Could you check a few things on this model? Use its own coordinates, in mm. Face numbers are marked on the shaded views. A direction names the side the tool comes from. Give positions to 0.01 mm unless a question says otherwise; leave off trailing zeros. Write each loop counter-clockwise with the first axis right and the second up, starting at its lowest first coordinate (ties: lowest second). Pieces come first, ordered by that corner, then holes. Notation, with made-up numbers: (60, 89) - (93, 89) arc R33 cw to (93, 121) - close; hole circle Ø8 at (36, 50.5). An arc over 180 degrees is marked (long way). Write item = value, one per line.
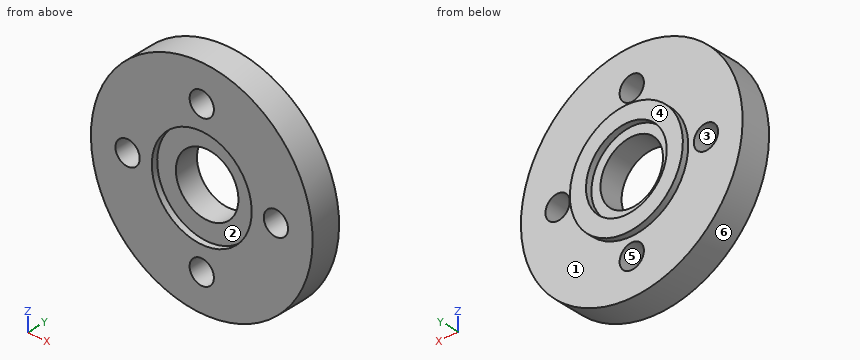
from build123d import *

# Parameters (mm, degrees)
CROQUIS_BASE_R             = 10.982321859
SALIENTE_EXTRUIR1_DEPTH    = 2.95
CORTAR_EXTRUIR1_DEPTH      = 16.809025486
CORTAR_EXTRUIR1_DEPTH_BACK = 16.809025486
CROQUIS_BASE_3_R           = 3
CROQUIS_BASE_3_R_2         = 1.202825727
CROQUIS_BASE_4_R           = 4.95
CORTAR_EXTRUIR2_DEPTH      = 0.6
CROQUIS2_R                 = 5.6
SALIENTE_EXTRUIR2_DEPTH    = 0.6
CROQUIS3_R                 = 3.1
CORTAR_EXTRUIR3_DEPTH      = 16.931895268
CROQUIS3_3_R               = 4
CORTAR_EXTRUIR4_DEPTH      = 0.6


with BuildPart() as part:
    # Croquis base → Saliente-Extruir1 (new body)
    with BuildSketch(Plane(origin=(0, 0, 0), x_dir=(1, 0, 0), z_dir=(0, 1, 0))):
        with Locations(Location((0, 0, 0), (0, 0, 270))):
            Circle(CROQUIS_BASE_R)
    extrude(amount=SALIENTE_EXTRUIR1_DEPTH)

    # Croquis base_3 → Cortar-Extruir1 (cut, two sides: drawn at the far end of the back side and taken through both)
    with BuildSketch(Plane(origin=(0, 0, 0), x_dir=(1, 0, 0), z_dir=(0, 1, 0)).offset(-CORTAR_EXTRUIR1_DEPTH_BACK)):
        with Locations(Location((0, 0, 0), (0, 0, 270))):
            Circle(CROQUIS_BASE_3_R)
        with Locations(Location((-7.35, 0, 0), (0, 0, 270))):
            Circle(CROQUIS_BASE_3_R_2)
        with Locations(Location((0, 7.35, 0), (0, 0, 270))):
            Circle(CROQUIS_BASE_3_R_2)
        with Locations(Location((7.35, 0, 0), (0, 0, 270))):
            Circle(CROQUIS_BASE_3_R_2)
        with Locations(Location((0, -7.35, 0), (0, 0, 270))):
            Circle(CROQUIS_BASE_3_R_2)
    extrude(amount=CORTAR_EXTRUIR1_DEPTH + CORTAR_EXTRUIR1_DEPTH_BACK, mode=Mode.SUBTRACT)

    # Croquis base_4 → Cortar-Extruir2 (cut)
    with BuildSketch(Plane(origin=(0, 0, 0), x_dir=(1, 0, 0), z_dir=(0, 1, 0))):
        with Locations(Location((0, 0, 0), (0, 0, 270))):
            Circle(CROQUIS_BASE_4_R)
    extrude(amount=CORTAR_EXTRUIR2_DEPTH, mode=Mode.SUBTRACT)

    # Croquis2 → Saliente-Extruir2 (add)
    with BuildSketch(Plane(origin=(0, 2.95, 0), x_dir=(1, 0, 0), z_dir=(0, 1, 0))):
        with Locations(Location((0, 0, 0), (0, 0, 270))):
            Circle(CROQUIS2_R)
    extrude(amount=SALIENTE_EXTRUIR2_DEPTH)

    # Croquis3 → Cortar-Extruir3 (cut, through all)
    with BuildSketch(Plane(origin=(0, 3.55, 0), x_dir=(1, 0, 0), z_dir=(0, 1, 0))):
        with Locations(Location((0, 0, 0), (0, 0, 270))):
            Circle(CROQUIS3_R)
    extrude(amount=-CORTAR_EXTRUIR3_DEPTH, mode=Mode.SUBTRACT)

    # Croquis3_3 → Cortar-Extruir4 (cut)
    with BuildSketch(Plane(origin=(0, 3.55, 0), x_dir=(1, 0, 0), z_dir=(0, 1, 0))):
        with Locations(Location((0, 0, 0), (0, 0, 270))):
            Circle(CROQUIS3_3_R)
    extrude(amount=-CORTAR_EXTRUIR4_DEPTH, mode=Mode.SUBTRACT)


solid = part.part
1. If we section it at D-D, the plane z = 7.35: Please give me the cut outline in (x, y), and give its area (3 significant figures).
Filled sheet:
outline = (-8.16, 0) - (-1.2, 0) - (-1.2, 2.95) - (-8.16, 2.95) - close; (1.2, 0) - (8.16, 0) - (8.16, 2.95) - (1.2, 2.95) - close
area = 41.0 mm2
2. I need wall thicknesses on line 1 (X direction, y = 1.25, z = 0); line 2 (X direction, y = 0.3, z = 0); line 3 (Y direction, x = -5.5, z = -2.5). Which ranges of each line are inside material? Lowest first, please.
Filled sheet:
line_1 = -10.98 to -8.55, -6.15 to -3.1, 3.1 to 6.15, 8.55 to 10.98
line_2 = -10.98 to -8.55, -6.15 to -4.95, 4.95 to 6.15, 8.55 to 10.98
line_3 = 0 to 2.95
3. Which directions (+Z, -Z, +X, -X, +Y, -Y) give clear straight access to the entire face, cutting with the end or side of a thin tool? Please do the marked faces 1, 2 and 3.
Filled sheet:
face_1 = +Y
face_2 = -Y
face_3 = +Y, -Y
4. Thinking about a two-plate mould opening in X: for the marked faces 4, 5 and 6, which applies, pulls with the +X half, pulls with the -X half, needs draft (parallel to the pull), parting line crosses it, or undercut?
Filled sheet:
face_4 = needs draft
face_5 = undercut
face_6 = parting line crosses it
5. For pin 1 (3 mm diameter, centred on x = -1, z = -2.5, fed in from -Y); pin 2 (3 mm diameter, centred on x = -7.35, z = 0, fed in from +Y); pin 3 (1 mm diameter, centred on x = -5.5, y = 2, fed in from -Z), each with a flat end and sliding along its axis, tell me the tip position at first contact or that it passes through.
Filled sheet:
pin_1 = 0.6
pin_2 = 2.95
pin_3 = -9.78
6. If we section it at C-C, the plane y = 2.3: Please give me the cut outline in (x, z), and give its area (3 significant figures).
Filled sheet:
outline = circle Ø21.96 at (0, 0); hole circle Ø2.41 at (-7.35, 0); hole circle Ø6.2 at (0, 0); hole circle Ø2.41 at (0, -7.35); hole circle Ø2.41 at (0, 7.35); hole circle Ø2.41 at (7.35, 0)
area = 331 mm2
7. If we section it at B-B, the plane z = 0: Please give me the cut outline in (x, y), and give its area (3 significant figures).
Filled sheet:
outline = (-10.98, 0) - (-8.55, 0) - (-8.55, 2.95) - (-10.98, 2.95) - close; (-6.15, 0) - (-4.95, 0) - (-4.95, 0.6) - (-3.1, 0.6) - (-3.1, 2.95) - (-4, 2.95) - (-4, 3.55) - (-5.6, 3.55) - (-5.6, 2.95) - (-6.15, 2.95) - close; (3.1, 0.6) - (4.95, 0.6) - (4.95, 0) - (6.15, 0) - (6.15, 2.95) - (5.6, 2.95) - (5.6, 3.55) - (4, 3.55) - (4, 2.95) - (3.1, 2.95) - close; (8.55, 0) - (10.98, 0) - (10.98, 2.95) - (8.55, 2.95) - close
area = 32.0 mm2
8. If we section it at A-A, the plane x = 0: Please give me the cut outline in (y, z).
Filled sheet:
outline = (0, -10.98) - (2.95, -10.98) - (2.95, -8.55) - (0, -8.55) - close; (0, -6.15) - (2.95, -6.15) - (2.95, -5.6) - (3.55, -5.6) - (3.55, -4) - (2.95, -4) - (2.95, -3.1) - (0.6, -3.1) - (0.6, -4.95) - (0, -4.95) - close; (0, 4.95) - (0.6, 4.95) - (0.6, 3.1) - (2.95, 3.1) - (2.95, 4) - (3.55, 4) - (3.55, 5.6) - (2.95, 5.6) - (2.95, 6.15) - (0, 6.15) - close; (0, 8.55) - (2.95, 8.55) - (2.95, 10.98) - (0, 10.98) - close
